from build123d import *

# Parameters (mm, degrees)
SKETCH1_R           = 12.5
BOSS_EXTRUDE1_DEPTH = 1
SKETCH2_R           = 1.675
SKETCH2_R_2         = 3.6
CUT_EXTRUDE1_DEPTH  = 1
BOSS_EXTRUDE3_START = -2
SKETCH3_R           = 13
SKETCH3_R_2         = 12.5
BOSS_EXTRUDE3_DEPTH = 2
SKETCH5_R           = 12.6
CUT_EXTRUDE2_DEPTH  = 1


with BuildPart() as part:
    # Sketch1 → Boss-Extrude1 (new body)
    with BuildSketch(Plane(origin=(0, 0, 0), x_dir=(1, 0, 0), z_dir=(0, 1, 0))):
        with Locations(Location((0, 0, 0), (0, 0, 270))):
            Circle(SKETCH1_R)
    extrude(amount=BOSS_EXTRUDE1_DEPTH)

    # Sketch2 → Cut-Extrude1 (cut)
    with BuildSketch(Plane(origin=(0, 1, 0), x_dir=(1, 0, 0), z_dir=(0, 1, 0))):
        with Locations(Location((0, 8.55, 0), (0, 0, 270))):
            Circle(SKETCH2_R)
        with Locations(Location((0, -8.55, 0), (0, 0, 270))):
            Circle(SKETCH2_R)
        with Locations(Location((0, 0, 0), (0, 0, 270))):
            Circle(SKETCH2_R_2)
    extrude(amount=-CUT_EXTRUDE1_DEPTH, mode=Mode.SUBTRACT)

    # Sketch3 → Boss-Extrude3 (add)
    with BuildSketch(Plane(origin=(0, 1, 0), x_dir=(1, 0, 0), z_dir=(0, 1, 0)).offset(BOSS_EXTRUDE3_START)):
        with Locations(Location((0, 0, 0), (0, 0, 270))):
            Circle(SKETCH3_R)
        with Locations(Location((0, 0, 0), (0, 0, 270))):
            Circle(SKETCH3_R_2, mode=Mode.SUBTRACT)
    extrude(amount=BOSS_EXTRUDE3_DEPTH)

    # Sketch5 → Cut-Extrude2 (cut)
    with BuildSketch(Plane.XZ.offset(1)):
        with Locations(Location((0, 0, 0), (0, 0, 270))):
            Circle(SKETCH5_R)
    extrude(amount=-CUT_EXTRUDE2_DEPTH, mode=Mode.SUBTRACT)


solid = part.part
Read the model definition and answer for the solid it produces. Units are mm, in the model's axes. A direction names the side the tool comes from. Round coordinates to 2 decimals unless told otherwise and drop trailing zeros. Loops run counter-clockwise (first coordinate to the right, second up) from the corner with the lowest first, then second, coordinate; pieces in that order, holes last.
Q1. Section B-B on x = 0 is taken. Write down the section's boundary in (y, z) (3 decimals), and give its area (3 significant figures).
Q2. Determine the mould class of faces 3 (the face through (-3, 1, 3)), 4 (the face through (-1.379, 0.507, 3.325)), 5 (the face through (-7.91, -0.014, -10.316)) for opening direction X: released by +X, released by -X, zero draft, split by the parting line, or undercut.
Q3. Section C-C on y = 0.7 is taken. Write down the section's boundary in (x, z) (3 decimals), and give its area (3 significant figures).
Q4. Which of the six approach directions +Z, -Z, +X, -X, +Y, -Y give full straight-line access (tool end or side, diameter ignored) to faces 1 (the face through (0.5, 0.51, 10.15)), 2 (the face through (-7.667, -0.507, 9.999))?
Q5. Section A-A on z = 0 is taken. Write down the section's boundary in (x, y), and give its area (3 significant figures).
Q6. Each of these flat-tipped pins is pushed along its axis until it touches: pin 1 (3 mm diameter, centred on x = -5, z = 7, fed in from -Y); pin 2 (1 mm diameter, centred on x = -7.5, y = 0, fed in from +Z). Where does it stop, or does it pass through?
Q7. Consider probe 1 along X at (y, z) = (-0.55, 0); probe 2 along Y at (x, z) = (4, 8.25); probe 3 along X at (y, z) = (0.5, 8.55) (3 decimals). Determine where each line is inside the solid, lowest interval first.
Q8. Section D-D on x = 6.75 is taken. Write down the section's boundary in (y, z).
Output:
1. outline: (-1, -13) - (1, -13) - (1, -10.225) - (0, -10.225) - (0, -12.6) - (-1, -12.6) - close; (-1, 12.6) - (0, 12.6) - (0, 10.225) - (1, 10.225) - (1, 13) - (-1, 13) - close; (0, -6.875) - (1, -6.875) - (1, -3.6) - (0, -3.6) - close; (0, 3.6) - (1, 3.6) - (1, 6.875) - (0, 6.875) - close
1. area: 12.9 mm2
2. face 3: zero draft
2. face 4: undercut
2. face 5: split by the parting line
3. outline: circle Ø26 at (0, 0); hole circle Ø7.2 at (0, 0); hole circle Ø3.35 at (0, -8.55); hole circle Ø3.35 at (0, 8.55)
3. area: 473 mm2
4. face 1: +Y, -Y
4. face 2: -Y
5. outline: (-13, -1) - (-12.6, -1) - (-12.6, 0) - (-3.6, 0) - (-3.6, 1) - (-13, 1) - close; (3.6, 0) - (12.6, 0) - (12.6, -1) - (13, -1) - (13, 1) - (3.6, 1) - close
5. area: 19.6 mm2
6. pin 1: stops at y = 0
6. pin 2: stops at z = 10.95
7. probe 1: x = -13 to -12.6, 12.6 to 13
7. probe 2: y = 0 to 1
7. probe 3: x = -9.793 to -1.675, 1.675 to 9.793
8. outline: (-1, -11.11) - (1, -11.11) - (1, 11.11) - (-1, 11.11) - (-1, 10.64) - (0, 10.64) - (0, -10.64) - (-1, -10.64) - close
